Autodesk Fusion 360 part; units mm, degrees
sketch "Sketch1" plane through (0, 0, 0) normal (0, 0, 1) x (1, 0, 0)
  line L0 (0, 0) -> (60, 0)
  line L1 (60, 0) -> (60, 30)
  line L2 (60, 30) -> (0, 30)
  line L3 (0, 30) -> (0, 0)
  dimension "d1" = 30
  dimension "d2" = 60
extrude "Extrude1" add sketch "Sketch1" along normal blind 12
sketch "Sketch2" plane through (60, 0, 0) normal (1, 0, 0) x (0, 1, 0)
  line L0 (0, 0) -> (30, 0)
  line L1 (30, 0) -> (30, 12)
  line L2 (30, 12) -> (0, 12)
  line L3 (0, 12) -> (0, 0)
  line L4 (0, 12) -> (4, 12)
  line L5 (4, 12) -> (4, 0)
  line L6 (4, 0) -> (0, 0)
  line L7 (0, 0) -> (0, 12)
  line L8 (30, 9.5242) -> (27, 9.5242)
  line L9 (27, 9.5242) -> (27, 2)
  line L10 (27, 2) -> (30, 2)
  line L11 (30, 2) -> (30, 9.5242)
extrude "Extrude2" add sketch "Sketch2" along normal blind 5 contours L0 L2 L3 L4 L5 L6 L7 | L1 L8 L9 L10 L11
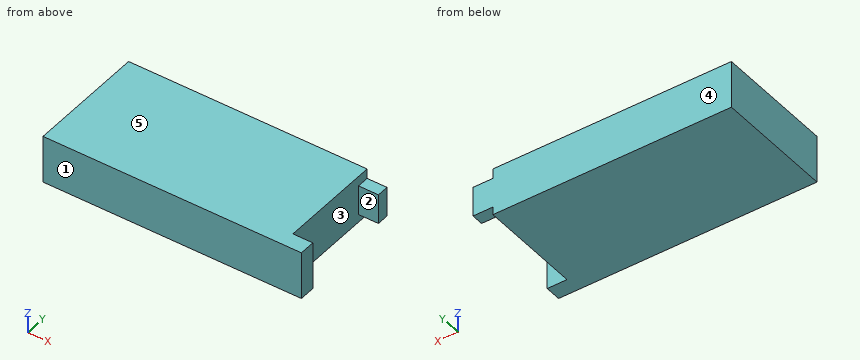
Verification items for the finished model (mm, model axes). Face numbers are marked on the shaded views. A direction names the side the tool comes from. Coordinates: 2 decimals unless noted, no trailing zeros. Order: outer loops, then holes, each group sorted by start corner. A loop starts at its lowest first (then second) coordinate and runs counter-clockwise, first axis right, second up. Notation, with made-up numbers: M 14,-25 L 45,-25 A17 ccw 45,-6 Z; hole C 8,-36 d10. An arc over 180 degrees is marked long. One line per item, written item: value. Start each with the question number.
Item 1: Mould release check, pull along Y, two halves, no side actions. Record for the marked faces 3, 4 and 5: pulls with the +Y half, pulls with the -Y half, needs draft (parallel to the pull), parting line crosses it, or undercut.
Item 2: Depth check by flat-ended pin: P1, Ø1.5, axis at x = 63, y = 28, coming from the -Z side; P2, Ø3.5, axis at y = 16, z = 6, coming from the +X side; P3, Ø3.5, axis at x = 62, y = 29, coming from the +Z side. Enter the tip coordinate at first touch or a pass-through.
Item 3: Sectioned sample at A-A on z = 5.25. Record the cut outline in (x, y).
Item 4: Sectioned sample at C-C on z = 11. Record the cut outline in (x, y).
Item 5: Thickness scan on probe 1 along X at (y, z) = (12.5, 7.5). Record the ranges inside material, lowest first.
Item 6: Access from +Z, -Z, +X, -X, +Y, -Y to the whole of each face (thin tool, end or side, straight path). Record for the marked faces 1 and 2.
Item 7: Sectioned sample at B-B on y = 10.75. Record the cut outline in (x, z), then the cut area to 3 significant figures.
Calculated:
1. face 3: undercut
1. face 4: pulls with the +Y half
1. face 5: needs draft
2. P1: z = 2
2. P2: x = 60
2. P3: z = 9.52
3. outline: M 0,0 L 65,0 L 65,4 L 60,4 L 60,27 L 65,27 L 65,30 L 0,30 Z
4. outline: M 0,0 L 65,0 L 65,4 L 60,4 L 60,30 L 0,30 Z
5. probe 1: 0 to 60
6. face 1: +Z, -Z, +X, -X, -Y
6. face 2: +Z, -Z, +X
7. outline: M 0,0 L 60,0 L 60,12 L 0,12 Z
7. area: 720 mm^2
